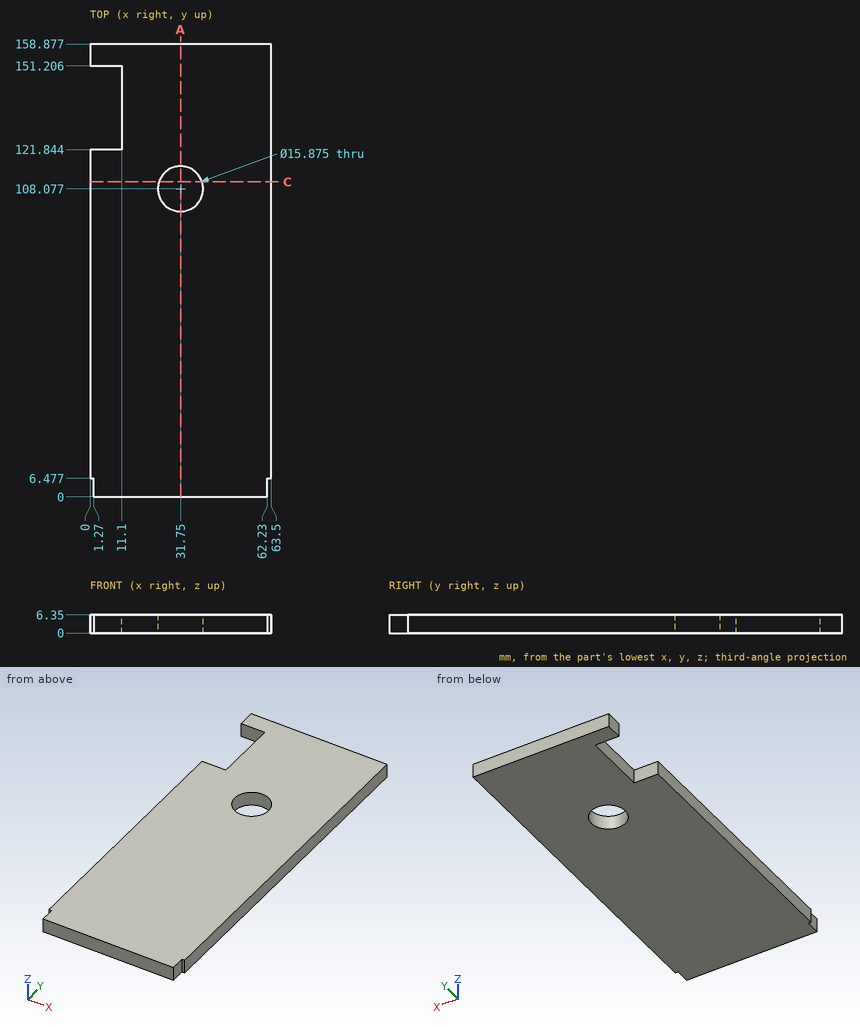
Print and shaded views of the part. All mm, measured from the part's lowest x, y and z. Coordinates: 2 decimals unless noted, no trailing zeros. Write each loop counter-clockwise with the first axis right and the second up, starting at its lowest first coordinate (ties: lowest second). Pieces come first, ordered by that corner, then holes. Notation, with made-up numbers: (-30.75, 2) - (-8.75, 2) arc R25 ccw to (-8.75, 34) - close; hole circle Ø10 at (-10, 75). An arc over 180 degrees is marked (long way). One line per question, with ' | ' between items. Start each with the question number.
Q1. Pin check, flat tips, straight feed: pin 1 (3 mm diameter, centred on y = 3.5, z = 4, fed in from -X); pin 2 (3 mm diameter, centred on x = 35, z = 4, fed in from -Y); pin 3 (1.4 mm diameter, centred on x = 63, z = 2, fed in from -Y); pin 4 (3 mm diameter, centred on y = 135, z = 2.5, fed in from -X). Stop position of each tip, or through.
Q2. Drill centre lines: line 1 (Y direction, x = 5.5, z = 5.5); line 2 (Y direction, x = 31.75, z = 2.75); line 3 (X direction, y = 142, z = 2.5). Where is each one in solid material? Low to high. Write a range as [from, to].
Q3. Cut at C-C, the plane y = 110.5. List the corners of the cut face in (x, z), then the cut area to 3 significant figures.
Q4. Cut at A-A, the plane x = 31.75. List the corners of the cut face in (y, z).
Answer below:
1) pin 1: x = 1.27 | pin 2: y = 0 | pin 3: y = 6.48 | pin 4: x = 11.1
2) line 1: [0, 121.84], [151.21, 158.88] | line 2: [0, 100.14], [116.01, 158.88] | line 3: [11.1, 63.5]
3) outline: (0, 0) - (24.19, 0) - (24.19, 6.35) - (0, 6.35) - close; (39.31, 0) - (63.5, 0) - (63.5, 6.35) - (39.31, 6.35) - close | area: 307 mm^2
4) outline: (0, 0) - (100.14, 0) - (100.14, 6.35) - (0, 6.35) - close; (116.01, 0) - (158.88, 0) - (158.88, 6.35) - (116.01, 6.35) - close
